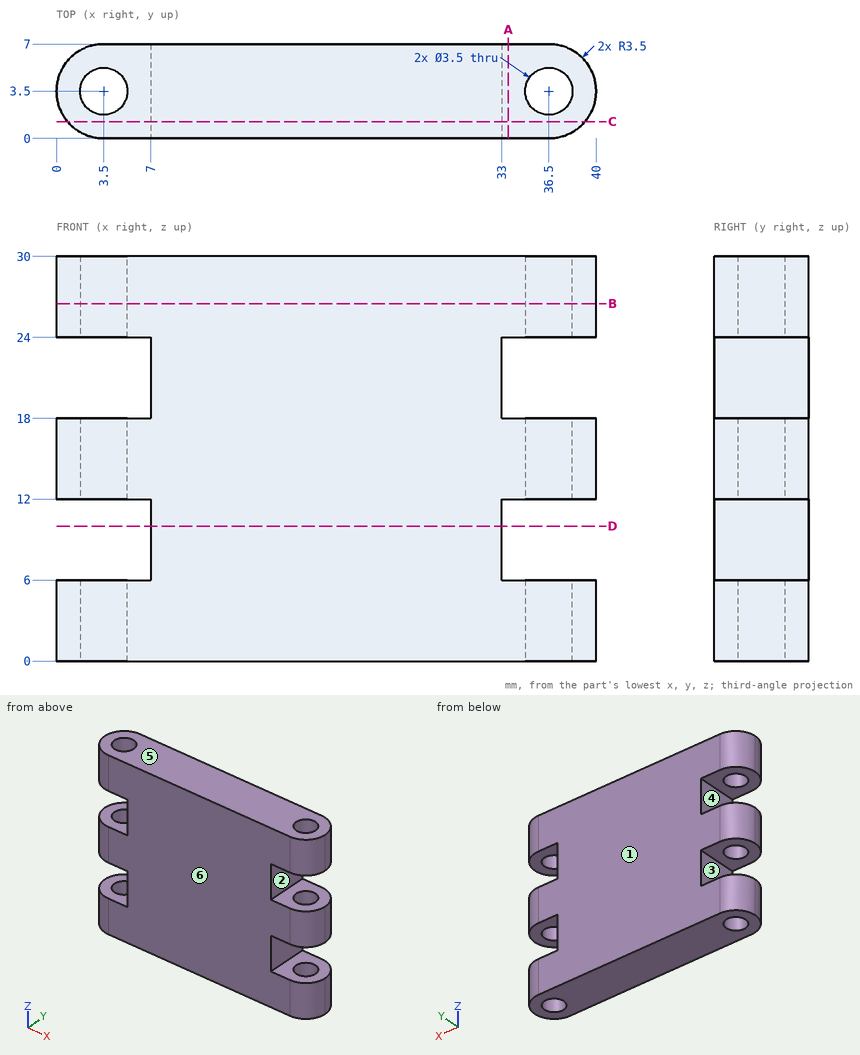
Here's the drawing with two shaded views (mm, measured from the low corner). I have some questions. A direction names the side the tool comes from. Give positions to 0.01 mm unless a question says otherwise; leave off trailing zeros. Loops run counter-clockwise (first coordinate to the right, second up) from the corner with the lowest first, then second, coordinate; pieces in that order, holes last. Notation, with made-up numbers: M 80,-17 L 117,-17 A24 cw 117,5 Z; hole C -15,77 d1. An arc over 180 degrees is marked long. Answer in a Markdown table with one row per item.
1. Thinking about a two-plate mould opening in Z: for the marked faces 4, 5 and 6, which applies, released by +Z, released by -Z, zero draft, split by the parting line, or undercut?
Taken from the geometry:
| item | result |
|---|---|
| face 4 | undercut |
| face 5 | released by +Z |
| face 6 | zero draft |
2. For pin 1 Ø3 at (x, y) = (3.5, 3.5) entering from -Z; pin 2 Ø1 at (y, z) = (1.5, 8) entering from +X, each with a flat end and sliding along its axis, tell me the tip position at first contact or that it passes through.
Taken from the geometry:
| item | result |
|---|---|
| pin 1 | passes through |
| pin 2 | stops at x = 33 |
3. Suppose I cut it at C-C on y = 1.25. Write out the boundary of the cut face in (x, z), plus the area to 3 significant figures.
Taken from the geometry:
| item | result |
|---|---|
| outline | M 0.82,0 L 39.18,0 L 39.18,6 L 33,6 L 33,12 L 39.18,12 L 39.18,18 L 33,18 L 33,24 L 39.18,24 L 39.18,30 L 0.82,30 L 0.82,24 L 7,24 L 7,18 L 0.82,18 L 0.82,12 L 7,12 L 7,6 L 0.82,6 Z |
| area | 1,000 mm² |
4. Suppose I cut it at D-D on z = 10. Write out the boundary of the cut face in (x, y).
Taken from the geometry:
| item | result |
|---|---|
| outline | M 7,0 L 33,0 L 33,7 L 7,7 Z |
5. Suppose I cut it at A-A on x = 33.5. Write out the boundary of the cut face in (y, z), plus the area to 3 significant figures.
Taken from the geometry:
| item | result |
|---|---|
| outline | M 0,0 L 7,0 L 7,6 L 0,6 Z; M 0,12 L 7,12 L 7,18 L 0,18 Z; M 0,24 L 7,24 L 7,30 L 0,30 Z |
| area | 126 mm² |
6. Suppose I cut it at B-B on z = 26.5. Write out the boundary of the cut face in (x, y).
Taken from the geometry:
| item | result |
|---|---|
| outline | M 3.5,0 L 36.5,0 A3.5 ccw 36.5,7 L 3.5,7 A3.5 ccw Z; hole C 3.5,3.5 d3.5; hole C 36.5,3.5 d3.5 |
7. Which directions (+Z, -Z, +X, -X, +Y, -Y) give clear straight access to the entire face, cutting with the end or side of a thin tool? Please do the marked faces 1, 2 and 3.
Taken from the geometry:
| item | result |
|---|---|
| face 1 | +Z, -Z, +X, -X, +Y |
| face 2 | +X, +Y, -Y |
| face 3 | -X, +Y, -Y |
8. If I drill on line 1 along X through (y, z) = (3.5, 4.7); line 2 along Z through (x, y) = (4.5, 6); line 3 along Y through (x, z) = (3.5, 2.65), over which ranges is the centre line in solid material (lowest first)?
Taken from the geometry:
| item | result |
|---|---|
| line 1 | x = 0 to 1.75, 5.25 to 34.75, 38.25 to 40 |
| line 2 | z = 0 to 6, 12 to 18, 24 to 30 |
| line 3 | y = 0 to 1.75, 5.25 to 7 |
